Source: CAD feature listing. Evaluate the final solid. Frame: model axes, mm. Face numbers are marked on the shaded views. Give positions to 0.01 mm unless a question says otherwise; leave off trailing zeros. Order: outer loops, then holes, each group sorted by start corner. A loop starts at its lowest first (then second) coordinate and runs counter-clockwise, first axis right, second up.
from build123d import *

# Parameters (mm, degrees)
F0_R     = 12.7
F1_DEPTH = 25.4


with BuildPart() as f1:
    # F0 (on Front) → F1 (new body)
    with BuildSketch(Plane.XZ):
        with BuildLine():
            ThreePointArc((37.607153, -6.108355), (37.976588, -3.064103), (38.1, 0))
            ThreePointArc((38.1, 0), (26.940768, 26.940768), (0, 38.1))
            ThreePointArc((0, 38.1), (-35.802072, -13.031564), (24.49118, -29.185477))
            Line((24.49118, -29.185477), (37.607153, -6.108355))
        make_face()
        Circle(F0_R, mode=Mode.SUBTRACT)
        with BuildLine():
            ThreePointArc((0, 38.1), (26.940768, 26.940768), (38.1, 0))
            ThreePointArc((38.1, 0), (37.976588, -3.064103), (37.607153, -6.108355))
            Line((37.607153, -6.108355), (72.515102, 55.311028))
            ThreePointArc((72.515102, 55.311028), (65.534173, 48.258733), (55.953582, 45.674062))
            Line((55.953582, 45.674062), (55.952777, 45.674062))
            ThreePointArc((55.952777, 45.674062), (38.250123, 57.688134), (42.875991, 78.576486))
            Line((42.875991, 78.576486), (0, 38.1))
        make_face()
        with BuildLine():
            ThreePointArc((24.49118, -29.185477), (33.123846, -18.826068), (37.607153, -6.108355))
            Line((37.607153, -6.108355), (24.49118, -29.185477))
        make_face()
        with BuildLine():
            ThreePointArc((75.003179, 64.724062), (63.495793, 82.217246), (42.875991, 78.576486))
            ThreePointArc((42.875991, 78.576486), (38.250123, 57.688134), (55.952777, 45.674062))
            Line((55.952777, 45.674062), (55.953582, 45.674062))
            ThreePointArc((55.953582, 45.674062), (65.534173, 48.258733), (72.515102, 55.311028))
            ThreePointArc((72.515102, 55.311028), (74.370659, 59.855907), (75.003179, 64.724062))
        make_face()
        with Locations((55.953179, 64.724062)):
            Circle(F0_R, mode=Mode.SUBTRACT)
    extrude(amount=F1_DEPTH)


solid = f1.part
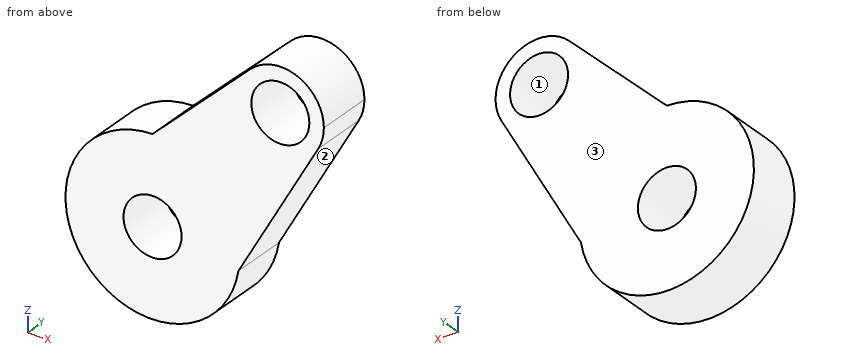
1) Section query C-C on x = 57. Output: boundary loops of the cut face in (y, z), and give its area (3 significant figures).
Checks:
outline: (-25.4, 28.01) - (0, 28.01) - (0, 52.07) - (-25.4, 52.07) - close; (-25.4, 77.38) - (0, 77.38) - (0, 83.75) - (-25.4, 83.75) - close
area: 773 mm2
2) Pull-direction query (X, two-part tool) for the marked faces 1, 2 and 3; classes: +X half, -X half, draft (parallel to the pull), parting line (faces both ways), or undercut.
Checks:
face 1: undercut
face 2: +X half
face 3: draft
3) Section query D-D on x = -29.5. Output: boundary loops of the cut face in (y, z), and give its area (3 significant figures).
Checks:
outline: (-25.4, -24.11) - (0, -24.11) - (0, 24.11) - (-25.4, 24.11) - close
area: 1,220 mm2
4) First-contact query: pin 1 Ø8 at (y, z) = (-14, 64) entering from -X; pin 2 Ø2 at (x, y) = (23, -5) entering from -Z; pin 3 Ø5 at (x, y) = (-26, -13) entering from -Z. Flat tips, straight axial feed; report the tip coordinate or a pass-through.
Checks:
pin 1: stops at x = 23.2
pin 2: stops at z = -31.11
pin 3: stops at z = -29.99
5) Ray query, L1, parallel to Z at x = 0, y = -9.25; L2, parallel to X at y = -14.25, z = 74.5; L3, parallel to Z at x = 53, y = -16.75. Return the intervals inside material, ascending.
Checks:
L1: z = -38.1 to -12.7, 12.7 to 38.1
L2: x = 38.56 to 47.85, 64.06 to 72.3
L3: z = 20.97 to 52.37, 77.08 to 83.54
6) Section query A-A on y = -5.5. Output: boundary loops of the cut face in (x, z), and give its area (3 significant figures).
Checks:
outline: (0, 38.1) arc R38.1 ccw (long way) to (24.49, -29.19) arc R38.1 ccw to (37.61, -6.11) - (72.52, 55.31) arc R19.05 ccw to (42.88, 78.58) - close; hole circle Ø25.4 at (0, 0); hole circle Ø25.4 at (55.95, 64.72)
area: 6,490 mm2
7) Section query B-B on z = 0. Output: boundary loops of the cut face in (x, y), and give its area (3 significant figures).
Checks:
outline: (-38.1, -25.4) - (-12.7, -25.4) - (-12.7, 0) - (-38.1, 0) - close; (12.7, -25.4) - (41.08, -25.4) - (41.08, 0) - (12.7, 0) - close
area: 1,370 mm2
